The model under review builds one solid part; all positions refer to its coordinate system, in mm. A direction names the side the tool comes from. Give positions to 0.01 mm unless a question says otherwise; leave off trailing zeros. Loops run counter-clockwise (first coordinate to the right, second up) from the corner with the lowest first, then second, coordinate; pieces in that order, holes last. Notation, with made-up numbers: (68, 17) - (98, 17) arc R24 cw to (98, 45) - close; hole circle Ø10 at (18.5, 55). An arc over 180 degrees is marked (long way). Answer as a JSON object with one key per item and string values.
from build123d import *

# Parameters (mm, degrees)
SKETCH_1_W          = 34
SKETCH_1_H          = 34
EXTRUDE_1_DEPTH     = 11
SKETCH_2_W          = 22
SKETCH_2_H          = 22
EXTRUDE_2_DEPTH     = 2
SKETCH_3_R          = 9
EXTRUDE_3_DEPTH     = 6
SKETCH_4_R          = 7
EXTRUDE_4_DEPTH     = 2
SKETCH_5_R          = 1.5
CUT_EXTRUDE_1_DEPTH = 34


with BuildPart() as part:
    # 草图1 → 凸台-拉伸1 (new body)
    with BuildSketch(Plane(origin=(0, 0, 0), x_dir=(1, 0, 0), z_dir=(0, 1, 0))):
        Rectangle(SKETCH_1_W, SKETCH_1_H)
    extrude(amount=EXTRUDE_1_DEPTH)

    # 草图2 → 凸台-拉伸2 (add)
    with BuildSketch(Plane(origin=(0, 11, 0), x_dir=(1, 0, 0), z_dir=(0, 1, 0))):
        Rectangle(SKETCH_2_W, SKETCH_2_H)
    extrude(amount=EXTRUDE_2_DEPTH)

    # 草图3 → 凸台-拉伸3 (add)
    with BuildSketch(Plane(origin=(0, 13, 0), x_dir=(1, 0, 0), z_dir=(0, 1, 0))):
        with Locations(Location((0, 0, 0), (0, 0, 270))):
            Circle(SKETCH_3_R)
    extrude(amount=EXTRUDE_3_DEPTH)

    # 草图4 → 凸台-拉伸4 (add)
    with BuildSketch(Plane(origin=(0, 19, 0), x_dir=(1, 0, 0), z_dir=(0, 1, 0))):
        with Locations(Location((0, 0, 0), (0, 0, 270))):
            Circle(SKETCH_4_R)
    extrude(amount=EXTRUDE_4_DEPTH)

    # 草图5 → 切除-拉伸1 (cut)
    with BuildSketch(Plane(origin=(17, 0, 0), x_dir=(0, 0, -1), z_dir=(1, 0, 0))):
        with Locations((0, 5.5)):
            Circle(SKETCH_5_R)
    extrude(amount=-CUT_EXTRUDE_1_DEPTH, mode=Mode.SUBTRACT)


solid = part.part
Q1. Clearance check with flat-ended pins moving along their axes: pin 1 Ø1 at (x, y) = (-4, 12.5) entering from -Z; pin 2 Ø1.6 at (x, y) = (1, 12) entering from +Z; pin 3 Ø6 at (x, z) = (1, -13.5) entering from +Y; pin 4 Ø10 at (x, z) = (4, -11.5) entering from -Y. State where each tip first meets the part, or that it passes through.
Results:
{"pin 1": "stops at z = -11", "pin 2": "stops at z = 11", "pin 3": "stops at y = 13", "pin 4": "stops at y = 0"}
Q2. Consider section B-B, the plane x = 0. State the section outline as (y, z) points, plus the area to 3 significant figures.
Results:
{"outline": "(0, -17) - (11, -17) - (11, -11) - (13, -11) - (13, -9) - (19, -9) - (19, -7) - (21, -7) - (21, 7) - (19, 7) - (19, 9) - (13, 9) - (13, 11) - (11, 11) - (11, 17) - (0, 17) - close; hole circle Ø3 at (5.5, 0)", "area": "547 mm^2"}
Q3. Consider section D-D, the plane y = 16.25. State the section outline as (x, z) points, plus the area to 3 significant figures.
Results:
{"outline": "circle Ø18 at (0, 0)", "area": "254 mm^2"}
Q4. To check wall thickness, follow probe 1 along Y at (x, z) = (-8, 0); probe 2 along Y at (x, z) = (1, 0); probe 3 along Y at (x, z) = (-7.5, 3). State the ranges of each line that lie inside material, in increasing order. Write a range as [from, to].
Results:
{"probe 1": "y = [0, 4], [7, 19]", "probe 2": "y = [0, 4], [7, 21]", "probe 3": "y = [0, 19]"}
Q5. For faces 1 (the face through (-7.3, 19, 0)), 2 (the face through (0, 12, 11)), 3 (the face through (-11, 12, 0)), list the 3-axis set-ups (+Z, -Z, +X, -X, +Y, -Y) from which the entire face can be reached by the end or side of a thin tool; tool diameter is ignored.
Results:
{"face 1": "+Y", "face 2": "+Z, +X, -X, +Y", "face 3": "+Z, -Z, -X, +Y"}
Q6. Consider section A-A, the plane z = 0. State the section outline as (x, y) points.
Results:
{"outline": "(-17, 0) - (17, 0) - (17, 4) - (-17, 4) - close; (-17, 7) - (17, 7) - (17, 11) - (11, 11) - (11, 13) - (9, 13) - (9, 19) - (7, 19) - (7, 21) - (-7, 21) - (-7, 19) - (-9, 19) - (-9, 13) - (-11, 13) - (-11, 11) - (-17, 11) - close"}
Q7. The part is to be moulded in two halves that separate along Z. For faces 4 (the face through (11, 12, 0)), 5 (the face through (2.703, 15.958, 8.584)), 6 (the face through (0, 4, 0)), say which applies: +Z half, -Z half, draft (parallel to the pull), parting line (faces both ways), or undercut.
Results:
{"face 4": "draft", "face 5": "parting line", "face 6": "undercut"}
Q8. Consider section C-C, the plane y = 5.5. State the section outline as (x, z) points.
Results:
{"outline": "(-17, -17) - (17, -17) - (17, -1.5) - (-17, -1.5) - close; (-17, 1.5) - (17, 1.5) - (17, 17) - (-17, 17) - close"}
